Autodesk Inventor part; units mm, degrees
ref_plane "MSC_PT1" through (7.5, 0, 0) normal (1, 0, 0) x (0, 1, 0)
ref_plane "MSC_PT2" through (0, 0, 0) normal (-1, 0, 0) x (0, -1, 0)
ref_plane "MSC_PF1" through (0, 0, 0) normal (1, 0, 0) x (0, 1, 0)
sketch "Sketch1" plane through (0, 0, 0) normal (1, 0, 0) x (0, 1, 0)
  line L0 (6.5, 3.7528) -> (6.5, -3.7528)
  line L1 (6.5, -3.7528) -> (0, -7.5056)
  line L2 (0, -7.5056) -> (-6.5, -3.7528)
  line L3 (-6.5, -3.7528) -> (-6.5, 3.7528)
  line L4 (-6.5, 3.7528) -> (0, 7.5056)
  line L5 (0, 7.5056) -> (6.5, 3.7528)
  circle A0 centre (0, 0) radius 6.5 construction
  dimension "d0" = 13
extrude "Extrusion1" add sketch "Sketch1" along normal blind 7.5
sketch "Sketch2" plane through (7.5, 0, 0) normal (1, 0, 0) x (0, 1, 0)
  line L0 (-6.5, 3.7528) -> (0, 7.5056)
  line L1 (0, -7.5056) -> (-6.5, -3.7528)
  line L2 (-6.5, 3.7528) -> (6.5, -3.7528) construction
  line L3 (-6.5, -3.7528) -> (6.5, 3.7528) construction
  point P0 (0, 0)
hole "Hole1" at (7.5, 0, 0) direction (-1, 0, 0) diameter 6.647 end through all
chamfer "Chamfer1" distance 0.625 angle 45 2 edges at (7.5, 0, 3.3235) (0, 0, 3.3235)
sketch "Sketch3" plane through (0, 0, 0) normal (0, 1, 0) x (-1, 0, 0)
  line L0 (-9.1715, 0) -> (2.5289, 0)
  line L1 (-5.7048, 0) -> (0.8574, 0)
  line L2 (-7.5, 0) -> (-7.5, -7.5056)
  line L3 (-7.5, -7.5056) -> (0, -7.5056)
  line L4 (0, -7.5056) -> (0, 0)
  line L5 (-7.5, -3.7528) -> (-7.5, -7.5056)
  line L6 (0, -3.7528) -> (0, -7.5056)
  line L7 (0, -7.5056) -> (-7.5, -7.5056)
  line L8 (-7.5, -6.5) -> (-6.9194, -7.5056)
  line L9 (-7.5, -7.5056) -> (-7.5, -6.5)
  line L10 (-7.5, -7.5056) -> (-6.9194, -7.5056)
  line L11 (0, -6.5) -> (-0.5806, -7.5056)
  line L12 (-0.5806, -7.5056) -> (0, -7.5056)
  line L13 (0, -7.5056) -> (0, -6.5)
  dimension "d32" = 6.5
  dimension "d33" = 30
revolve "Revolution1" cut sketch "Sketch3" angle 360 about axis through (0, 0, 0) along (-1, 0, 0) contours L8 L3 L2 | L4 L3 L11
ref_plane "MSC_PT1" through (7.5, 0, 0) normal (1, 0, 0) x (0, 1, 0)
ref_plane "MSC_PT2" through (0, 0, 0) normal (-1, 0, 0) x (0, -1, 0)
ref_plane "MSC_PF1" through (0, 0, 0) normal (1, 0, 0) x (0, 1, 0)
equation "\"d0\" = Smax"
equation "\"d1\" = Mmax"
equation "\"d10\" = 0.5 * PTC"
equation "\"d32\" = 0.5 * Smax"
equation "\"NND\" = 8"
equation "\"Smax\" = 13"
equation "\"Mmax\" = 7.5"
equation "\"PTC\" = 1.25"
equation "\"THREADDIA\" = NND"
equation "\"TEMPLATE\" = 1.2345"
properties part number "ANSI B18.2.4.2M - M8x1.25" material "Steel, Mild"
Verification items for the finished model (mm, model axes). Give positions to 0.01 mm unless a question says otherwise; leave off trailing zeros. Order: outer loops, then holes, each group sorted by start corner. A loop starts at its lowest first (then second) coordinate and runs counter-clockwise, first axis right, second up. Notation, with made-up numbers: M -11,-4 L 11,-4 A26 cw 11,14 Z; hole C -3.75,23.25 d3. An arc over 180 degrees is marked long. Answer in a Markdown table with one row per item. Add a question column.
Item 1: Gauge pin test, flat ends, axial feed: pin 1 (2 mm diameter, centred on x = 3, y = 3.5, fed in from +Z); pin 2 (2 mm diameter, centred on x = 6, y = 1.5, fed in from -Z); pin 3 (3 mm diameter, centred on x = 6, z = -5.5, fed in from -Y). Record the tip position at first contact, or that the pin passes through.
Item 2: Scan lines: probe 1 along Y at (x, z) = (3, 0); probe 2 along Z at (x, y) = (6, 3); probe 3 along Y at (x, z) = (2.25, -2.5). Record each from-to range of solid material in increasing order. Write a range as from..to.
Item 3: Section check A-A, the plane x = 4.75. Enter the section's corners in (y, z).
Item 4: Mould release check, pull along Z, two halves, no side actions. Record for faces 1 (the flat face through (7.5, 3, -3)), 2 (the flat face through (3.7, -3.3, 5.6)), 3 (the cylindrical face through (3.71, 1.27, -3.07)): released by +Z, released by -Z, zero draft, split by the parting line, or undercut.
Filled sheet:
| question | item | result |
|---|---|---|
| 1 | pin 1 | stops at z = 6.06 |
| 1 | pin 2 | stops at z = -7.22 |
| 1 | pin 3 | stops at y = -6.07 |
| 2 | probe 1 | y = -6.5..-3.32, 3.32..6.5 |
| 2 | probe 2 | z = -5.77..-1.43, 1.43..5.77 |
| 2 | probe 3 | y = -6.5..-2.19, 2.19..6.5 |
| 3 | outline | M -6.5,-3.75 L 0,-7.51 L 6.5,-3.75 L 6.5,3.75 L 0,7.51 L -6.5,3.75 Z; hole C 0,0 d6.65 |
| 4 | face 1 | zero draft |
| 4 | face 2 | released by +Z |
| 4 | face 3 | undercut |
